Read the model definition and answer for the solid it produces. Units are mm, in the model's axes. A direction names the side the tool comes from. Coordinates: 2 decimals unless noted, no trailing zeros. Loops run counter-clockwise (first coordinate to the right, second up) from the corner with the lowest first, then second, coordinate; pieces in that order, holes last. Notation, with made-up numbers: (41, -19.75) -> (70, -19.75) arc R21 ccw to (70, -4.75) -> close; hole circle Ø1 at (29, 7). An arc over 180 degrees is marked (long way). Answer as CSV lines item,"result".
```python
from build123d import *

# Parameters (mm, degrees)
SKETCH1_R           = 12.5
BOSS_EXTRUDE1_DEPTH = 3


with BuildPart() as part:
    # Sketch1 → Boss-Extrude1 (new body)
    with BuildSketch(Plane.XY):
        with BuildLine():
            Line((-15, 27.5), (15, 27.5))
            Line((15, 27.5), (15, 30.5))
            Line((15, 30.5), (45, 30.5))
            Line((45, 30.5), (45, 27.5))
            ThreePointArc((45, 27.5), (39.142135624, 13.357864376), (25, 7.5))
            ThreePointArc((25, 7.5), (19.696699141, 5.303300859), (17.5, 0))
            ThreePointArc((17.5, 0), (0, -17.5), (-17.5, 0))
            ThreePointArc((-17.5, 0), (-19.696699141, 5.303300859), (-25, 7.5))
            ThreePointArc((-25, 7.5), (-39.142135624, 13.357864376), (-45, 27.5))
            Line((-45, 27.5), (-45, 30.5))
            Line((-45, 30.5), (-15, 30.5))
            Line((-15, 30.5), (-15, 27.5))
        make_face()
        Circle(SKETCH1_R, mode=Mode.SUBTRACT)
    extrude(amount=BOSS_EXTRUDE1_DEPTH)


solid = part.part
```
Q1. Find the intervals of material crossed by probe 1 along Y at (x, z) = (0, 1.8); probe 2 along Y at (x, z) = (25, 0.4); probe 3 along X at (y, z) = (-8, 1.75), in increasing order. Write a range as [from, to].
Results:
probe 1,"y = [-17.5, -12.5], [12.5, 27.5]"
probe 2,"y = [7.5, 30.5]"
probe 3,"x = [-15.56, -9.6], [9.6, 15.56]"
Q2. Given pin 1 Ø3 at (x, y) = (-9.5, 21) entering from -Z, flat-ended and moving along its own axis, determine where the tip first touches the part or whether it passes through.
Results:
pin 1,"stops at z = 0"
Q3. A cutting plane is placed at B-B, the plane z = 1.95. Write down the section's boundary in (x, y), and give its area (3 significant figures).
Results:
outline,"(-45, 27.5) arc R20 ccw to (-25, 7.5) arc R7.5 cw to (-17.5, 0) arc R17.5 ccw to (17.5, 0) arc R7.5 cw to (25, 7.5) arc R20 ccw to (45, 27.5) -> (45, 30.5) -> (15, 30.5) -> (15, 27.5) -> (-15, 27.5) -> (-15, 30.5) -> (-45, 30.5) -> close; hole circle Ø25 at (0, 0)"
area,"2,090 mm²"
Q4. For a pull along Y with two mould halves and no side action, classify faces 1 (the face through (-30, 30.5, 1)), 2 (the face through (-45, 29, 1)), 3 (the face through (-38.986, 13.203, 1.479)), 4 (the face through (11.923, 3.755, 1.479)) as pulls with the +Y half, pulls with the -Y half, needs draft (parallel to the pull), parting line crosses it, or undercut.
Results:
face 1,"pulls with the +Y half"
face 2,"needs draft"
face 3,"pulls with the -Y half"
face 4,"undercut"
Q5. A cutting plane is placed at D-D, the plane x = -19. Write down the section's boundary in (y, z), and give its area (3 significant figures).
Results:
outline,"(4.5, 0) -> (30.5, 0) -> (30.5, 3) -> (4.5, 3) -> close"
area,"78.0 mm²"
Q6. For faces 5 (the face through (0, 27.5, 1)), 6 (the face through (1, 18, 3)), determine the directions among +Z, -Z, +X, -X, +Y, -Y from which every point of the face is accessible in a straight line to the end or side of a thin tool.
Results:
face 5,"+Z, -Z, +Y"
face 6,"+Z, +X, -X, +Y, -Y"
Q7. A cutting plane is placed at C-C, the plane y = -5.5. Write down the section's boundary in (x, z).
Results:
outline,"(-16.61, 0) -> (-11.22, 0) -> (-11.22, 3) -> (-16.61, 3) -> close; (11.22, 0) -> (16.61, 0) -> (16.61, 3) -> (11.22, 3) -> close"
Q8. A cutting plane is placed at A-A, the plane x = 0. Write down the section's boundary in (y, z), and give its area (3 significant figures).
Results:
outline,"(-17.5, 0) -> (-12.5, 0) -> (-12.5, 3) -> (-17.5, 3) -> close; (12.5, 0) -> (27.5, 0) -> (27.5, 3) -> (12.5, 3) -> close"
area,"60.0 mm²"
